Read the model definition and answer for the solid it produces. Units are mm, in the model's axes. A direction names the side the tool comes from. Give positions to 0.01 mm unless a question says otherwise; leave off trailing zeros. Order: outer loops, then holes, each group sorted by start corner. A loop starts at its lowest first (then second) coordinate and runs counter-clockwise, first axis right, second up. Notation, with made-up numbers: M 8.25,8.25 L 56.25,8.25 A11 cw 56.25,28.25 Z; hole C -13,8 d6. An arc over 180 degrees is marked long. Write item = value, one per line. Start each with the question number.
from build123d import *

# Parameters (mm, degrees)
SKETCH1_R           = 3.3
BOSS_EXTRUDE1_DEPTH = 8
SKETCH2_R           = 1.2
BOSS_EXTRUDE2_DEPTH = 5
SKETCH3_R           = 2.05
CUT_EXTRUDE1_DEPTH  = 2
FILLET1_R           = 0.5
FILLET2_R           = 1


with BuildPart() as part:
    # Sketch1 → Boss-Extrude1 (new body)
    with BuildSketch(Plane(origin=(0, 0, 0), x_dir=(1, 0, 0), z_dir=(0, 1, 0))):
        with Locations(Location((0, 0, 0), (0, 0, 270))):
            Circle(SKETCH1_R)
    extrude(amount=BOSS_EXTRUDE1_DEPTH)

    # Sketch2 → Boss-Extrude2 (add)
    with BuildSketch(Plane(origin=(0, 8, 0), x_dir=(1, 0, 0), z_dir=(0, 1, 0))):
        with BuildLine():
            Line((-9.841666667, 4.979367151), (-1.091666667, 6.458387097))
            ThreePointArc((-1.091666667, 6.458387097), (0, 6.55), (1.091666667, 6.458387097))
            Line((1.091666667, 6.458387097), (9.841666667, 4.979367151))
            ThreePointArc((9.841666667, 4.979367151), (14.05, 0), (9.841666667, -4.979367151))
            Line((9.841666667, -4.979367151), (1.091666667, -6.458387097))
            ThreePointArc((1.091666667, -6.458387097), (0, -6.55), (-1.091666667, -6.458387097))
            Line((-1.091666667, -6.458387097), (-9.841666667, -4.979367151))
            ThreePointArc((-9.841666667, -4.979367151), (-14.05, 0), (-9.841666667, 4.979367151))
        make_face()
        with Locations(Location((-9, 0, 0), (0, 0, 270))):
            Circle(SKETCH2_R, mode=Mode.SUBTRACT)
        with Locations(Location((9, 0, 0), (0, 0, 270))):
            Circle(SKETCH2_R, mode=Mode.SUBTRACT)
    extrude(amount=BOSS_EXTRUDE2_DEPTH)

    # Sketch3 → Cut-Extrude1 (cut)
    with BuildSketch(Plane(origin=(0, 13, 0), x_dir=(1, 0, 0), z_dir=(0, 1, 0))):
        with Locations(Location((-9, 0, 0), (0, 0, 270))):
            Circle(SKETCH3_R)
        with Locations(Location((9, 0, 0), (0, 0, 270))):
            Circle(SKETCH3_R)
    extrude(amount=-CUT_EXTRUDE1_DEPTH, mode=Mode.SUBTRACT)

    # Fillet1
    fillet1_edges = [part.edges().sort_by_distance(p)[0] for p in [
        (5.466666667, 8, 5.718877124),
        (14.05, 8, 0),
        (5.466666667, 8, -5.718877124),
        (0, 8, -6.55),
        (-5.466666667, 8, -5.718877124),
        (-9, 13, -2.05),
        (9, 13, -2.05),
        (-14.05, 8, 0),
        (-5.466666667, 8, 5.718877124),
        (0, 8, 6.55),
    ]]
    fillet(fillet1_edges, radius=FILLET1_R)

    # Fillet2
    fillet2_edges = [part.edges().sort_by_distance(p)[0] for p in [
        (-14.05, 13, 0),
        (-5.466666667, 13, 5.718877124),
        (0, 13, 6.55),
        (5.466666667, 13, 5.718877124),
        (14.05, 13, 0),
        (5.466666667, 13, -5.718877124),
        (0, 13, -6.55),
        (-5.466666667, 13, -5.718877124),
    ]]
    fillet(fillet2_edges, radius=FILLET2_R)


solid = part.part
1) For a pull along X with two mould halves and no side action, classify faces 1 (the face through (-10.17, 9.48, -0.26)), 2 (the face through (-5.5, 8.14, 5.56)), 3 (the face through (5.41, 10.23, -5.73)) as pulls with the +X half, pulls with the -X half, needs draft (parallel to the pull), parting line crosses it, or undercut.
2) Find the intervals of material crossed by probe 1 along Y at (x, z) = (1.5, 5.5); probe 2 along Y at (x, z) = (-7.75, 0); probe 3 along X at (y, z) = (4.5, -2.25), in increasing order. Write a range as [from, to].
3) For faces 4 (the face through (-10, 11, 1)), 5 (the face through (7.83, 9.48, -0.26)), 6 (the face through (-2.008, 3.944, -2.619)), determine the directions among +Z, -Z, +X, -X, +Y, -Y from which every point of the face is accessible in a straight line to the end or side of a thin tool.
4) Find section A-A on x = 0. Determine the outline of the cut face in (y, z).
5) Each of these flat-tipped pins is pushed along its axis until it touches: P1, Ø1.2, axis at x = -9, z = 1, coming from the +Y side; P2, Ø4, axis at y = 4, z = 5, coming from the +X side; P3, Ø1, axis at x = -10, y = 9, coming from the -Z side. Where does it stop, or does it pass through?
6) Find section C-C on y = 4.25. Determine the outline of the cut face in (x, z), plus the area to 3 significant figures.
7) Find section B-B on y = 10.25. Determine the outline of the cut face in (x, z), plus the area to 3 significant figures.
Numbers:
q1.face_1 = undercut
q1.face_2 = pulls with the -X half
q1.face_3 = pulls with the +X half
q2.probe_1 = [8, 12.99]
q2.probe_2 = [8, 11]
q2.probe_3 = [-2.41, 2.41]
q3.face_4 = +Y
q3.face_5 = +Y, -Y
q3.face_6 = -Y
q4.outline = M 0,-3.3 L 8,-3.3 L 8,-6.05 A0.5 ccw 8.5,-6.55 L 12,-6.55 A1 ccw 13,-5.55 L 13,5.55 A1 ccw 12,6.55 L 8.5,6.55 A0.5 ccw 8,6.05 L 8,3.3 L 0,3.3 Z
q5.P1 = 11
q5.P2 = 1.37
q5.P3 = -5.04
q6.outline = C 0,0 d6.6
q6.area = 34.2 mm2
q7.outline = M -9.84,-4.98 L -1.09,-6.46 A6.55 ccw 1.09,-6.46 L 9.84,-4.98 A5.05 ccw 9.84,4.98 L 1.09,6.46 A6.55 ccw -1.09,6.46 L -9.84,4.98 A5.05 ccw Z; hole C -9,0 d2.4; hole C 9,0 d2.4
q7.area = 283 mm2
